Input: dimensioned drawing with shaded views. Units: mm. Origin: part minimum x, y, z. A direction names the side the tool comes from. Round coordinates to 2 decimals unless told otherwise and drop trailing zeros. Loops run counter-clockwise (first coordinate to the right, second up) from the corner with the lowest first, then second, coordinate; pieces in that order, holes last.
Item 1: Section query A-A on x = 116. Return loops of the section in (y, z).
Item 2: First-contact query: P1, Ø1.5, axis at y = 123.5, z = 110.5, coming from the +X side; P2, Ø4, axis at y = 166.5, z = 104, coming from the -X side; P3, Ø25, axis at x = 115, z = 125, coming from the +Y side. Flat tips, straight axial feed; report the tip coordinate or a pass-through.
Item 3: Pull-direction query (Z, two-part tool) for the marked faces 4, 5, 6 and 7; classes: released by +Z, released by -Z, zero draft, split by the parting line, or undercut.
Item 4: Section query B-B on y = 225. Return loops of the section in (x, z), then the cut area to 3 significant figures.
Item 5: Section query D-D on x = 181. Return loops of the section in (y, z).
Item 6: Ray query, L1, parallel to Y at x = 125, z = 175.75; L2, parallel to Z at x = 149.5, y = 240; L3, parallel to Y at x = 125, z = 79.25. Return the intervals inside material, ascending.
Item 7: Access query for the marked faces 1, 2 and 3. Directions: +Z, -Z, +X, -X, +Y, -Y. A direction counts if a zero-diameter tool reaches every point of the face in a straight line with its end or side. Return the directions, or none.
Item 8: Section query C-C on z = 158.5. Return loops of the section in (x, y), then the cut area to 3 significant figures.
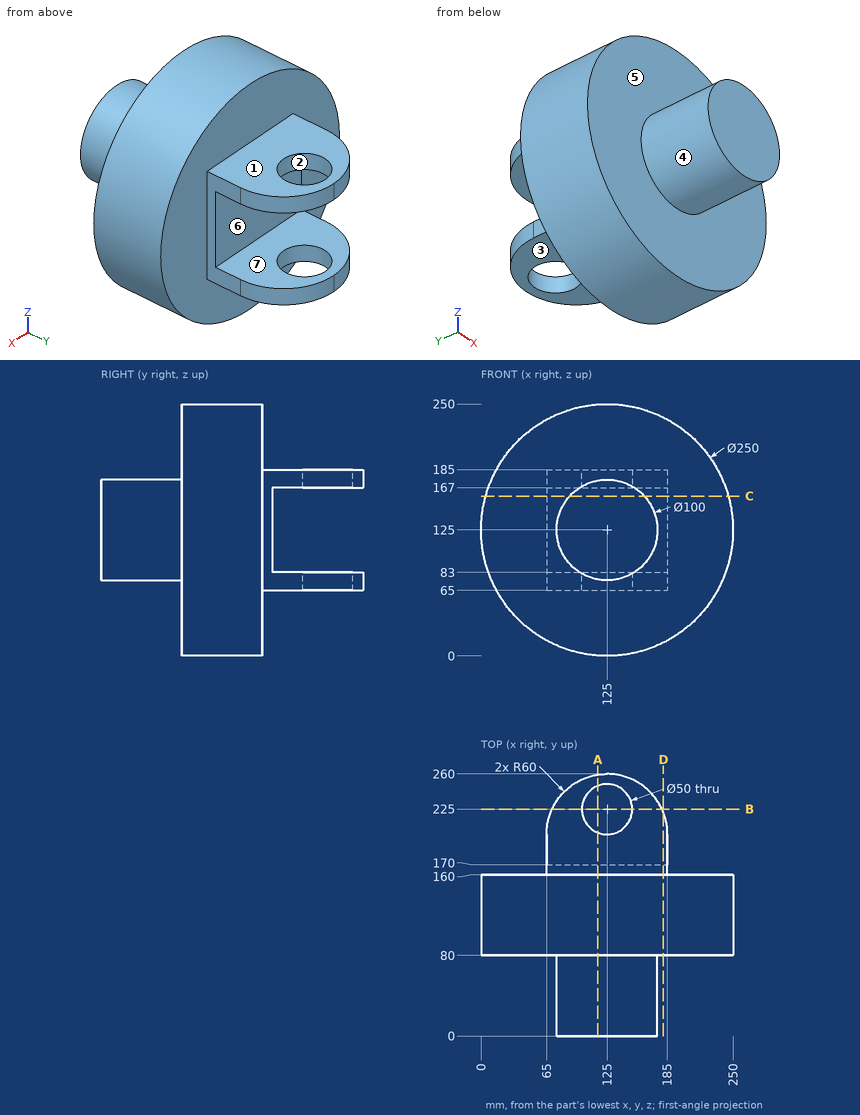
Data:
1. outline: (0, 75.82) - (80, 75.82) - (80, 0.32) - (160, 0.32) - (160, 65) - (201.68, 65) - (201.68, 83) - (170, 83) - (170, 167) - (201.68, 167) - (201.68, 185) - (160, 185) - (160, 249.68) - (80, 249.68) - (80, 174.18) - (0, 174.18) - close; (248.32, 65) - (259.32, 65) - (259.32, 83) - (248.32, 83) - close; (248.32, 167) - (259.32, 167) - (259.32, 185) - (248.32, 185) - close
2. P1: stops at x = 249.24
2. P2: stops at x = 65
2. P3: stops at y = 170
3. face 4: split by the parting line
3. face 5: zero draft
3. face 6: undercut
3. face 7: undercut
4. outline: (70.46, 65) - (100, 65) - (100, 83) - (70.46, 83) - close; (70.46, 167) - (100, 167) - (100, 185) - (70.46, 185) - close; (150, 65) - (179.54, 65) - (179.54, 83) - (150, 83) - close; (150, 167) - (179.54, 167) - (179.54, 185) - (150, 185) - close
4. area: 2,130 mm2
5. outline: (80, 13.25) - (160, 13.25) - (160, 65) - (221.54, 65) - (221.54, 83) - (170, 83) - (170, 167) - (221.54, 167) - (221.54, 185) - (160, 185) - (160, 236.75) - (80, 236.75) - close
6. L1: y = 80 to 200, 250 to 260
6. L2: z = 65 to 83, 167 to 185
6. L3: y = 0 to 200, 250 to 260
7. face 1: +Z, +X, -X, +Y
7. face 2: +Z, -Z
7. face 3: -Z, +X, -X, +Y
8. outline: (4.57, 80) - (87.88, 80) - (87.88, 0) - (162.12, 0) - (162.12, 80) - (245.43, 80) - (245.43, 160) - (185, 160) - (185, 170) - (65, 170) - (65, 160) - (4.57, 160) - close
8. area: 26,400 mm2
